from build123d import *

# Parameters (mm, degrees)
SKETCH_1_W                  = 20
SKETCH_1_H                  = 20
EXTRUDE_1_DEPTH             = 5
SKETCH_2_W                  = 5
SKETCH_2_H                  = 20
EXTRUDE_2_DEPTH             = 35
HOLE_WIZARD_M3_1_AT_2_COUNT = 2
HOLE_WIZARD_M3_1_AT_2_PITCH = 12
SKETCH_5_W                  = 5
SKETCH_5_H                  = 20
EXTRUDE_3_DEPTH             = 7


with BuildPart() as part:
    # 草圖1 → 填料-伸長1 (new body)
    with BuildSketch(Plane(origin=(0, 0, 0), x_dir=(1, 0, 0), z_dir=(0, 1, 0))):
        Rectangle(SKETCH_1_W, SKETCH_1_H)
    extrude(amount=EXTRUDE_1_DEPTH)

    # 草圖2 → 填料-伸長2 (add)
    with BuildSketch(Plane.XZ):
        Rectangle(SKETCH_2_W, SKETCH_2_H)
    extrude(amount=EXTRUDE_2_DEPTH)

    # 草圖4 → M3 螺紋孔1 (revolve, cut)
    with BuildSketch(Plane(origin=(0, -18, 10), x_dir=(0, -1, 0), z_dir=(1, 0, 0))):
        Polygon((0, 0), (0, 7.251075774), (1.25, 6.5), (1.25, 0), align=None)
    hole_wizard_m3_1 = revolve(axis=Axis((0, -18, 16.35), (0, 0, -1)), mode=Mode.SUBTRACT)

    # M3 螺紋孔1 at 2: M3 螺紋孔1 ×2
    with Locations(*[(0, -i * HOLE_WIZARD_M3_1_AT_2_PITCH, 0) for i in range(1, HOLE_WIZARD_M3_1_AT_2_COUNT)]):
        add(hole_wizard_m3_1, mode=Mode.SUBTRACT)

    # 鏡射1: M3 螺紋孔1 across plane
    add(hole_wizard_m3_1.mirror(Plane.XY), mode=Mode.SUBTRACT)

    # 鏡射1 copy 1 sketch → 鏡射1 copy 1 (revolve, cut)
    with BuildSketch(Plane(origin=(0, -30, -10), x_dir=(0, -1, 0), z_dir=(1, 0, 0))):
        Polygon((0, 0), (0, -7.251075774), (1.25, -6.5), (1.25, 0), align=None)
    revolve(axis=Axis((0, -30, -16.35), (0, 0, -1)), mode=Mode.SUBTRACT)

    # 草圖5 → 填料-伸長3 (add)
    with BuildSketch(Plane.XZ.offset(35)):
        Rectangle(SKETCH_5_W, SKETCH_5_H)
    extrude(amount=EXTRUDE_3_DEPTH)


solid = part.part
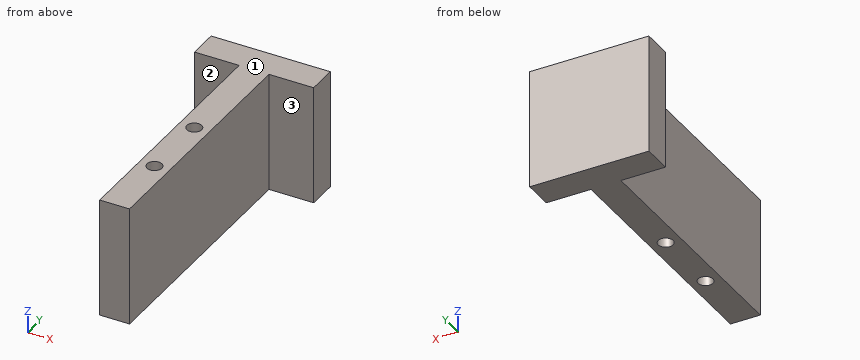
Read the model definition and answer for the solid it produces. Units are mm, in the model's axes. Face numbers are marked on the shaded views. A direction names the side the tool comes from. Round coordinates to 2 decimals unless told otherwise and drop trailing zeros. Order: outer loops, then holes, each group sorted by start corner. A loop starts at its lowest first (then second) coordinate and runs counter-clockwise, first axis right, second up. Notation, with made-up numbers: (60, 54) - (89, 54) arc R21 cw to (89, 80) - close; hole circle Ø6 at (-13, 40.5). An arc over 180 degrees is marked (long way). Use one line per item in the form item = value. Start each with the question number.
(1) Find the intervals of material crossed by line 1 along Y through (x, z) = (0, 6); line 2 along X through (y, z) = (-30, 7.25); line 3 along X through (y, z) = (-34.5, -2.75), in increasing order. Write a range as from..to.
(2) Flat-ended cylindrical pins translate along their axes: pin 1 Ø3 at (y, z) = (-33, -4.5) entering from +X; pin 2 Ø6 at (x, y) = (6, -19.5) entering from -Z; pin 3 Ø1.5 at (x, y) = (0, -18) entering from +Z; pin 4 Ø6 at (y, z) = (-21, -2) entering from -X. Find the tip coordinate at first contact, or state that the pin passes through.
(3) For the marked faces 1, 2 and 3, determine the directions among +Z, -Z, +X, -X, +Y, -Y from which every point of the face is accessible in a straight line to the end or side of a thin tool.
(4) The part is cut by section B-B (x = 5.5). Give the vertices of the cut face in (y, z).
(5) The part is cut by section A-A (z = -9). Give the vertices of the cut face in (x, y), then the cut area to 3 significant figures.
(6) The part is cut by section C-C (y = -36). Give the vertices of the cut face in (x, z), then the cut area to 3 significant figures.
Checked values:
q1.line_1 = -42..-31.25, -28.75..-19.25, -16.75..5
q1.line_2 = -2.5..-1.25, 1.25..2.5
q1.line_3 = -2.5..2.5
q2.pin_1 = 2.5
q2.pin_2 = through
q2.pin_3 = 3.2
q2.pin_4 = -2.5
q3.face_1 = +Z, +X, -X, +Y, -Y
q3.face_2 = +Z, -Z, -X, -Y
q3.face_3 = +Z, -Z, +X, -Y
q4.outline = (0, -10) - (5, -10) - (5, 10) - (0, 10) - close
q5.outline = (-10, 0) - (-2.5, 0) - (-2.5, -42) - (2.5, -42) - (2.5, 0) - (10, 0) - (10, 5) - (-10, 5) - close; hole circle Ø2.5 at (0, -30); hole circle Ø2.5 at (0, -18)
q5.area = 300 mm^2
q6.outline = (-2.5, -10) - (2.5, -10) - (2.5, 10) - (-2.5, 10) - close
q6.area = 100 mm^2
